from build123d import *

# Parameters (mm, degrees)
SZKIC2_W                    = 25.000000373
SZKIC2_H                    = 24
SZKIC2_R                    = 1.05
DODANIE_WYCI_GNI_CIE1_DEPTH = 5
SZKIC3_R                    = 1.05
WYTNIJ_WYCI_GNI_CIE1_DEPTH  = 36.134524248
SZKIC4_W                    = 2.5
SZKIC4_H                    = 6.5
SZKIC4_H_2                  = 12.5
WYTNIJ_WYCI_GNI_CIE2_DEPTH  = 36.134524248
ZAOKR_GLENIE5_R             = 2.5


with BuildPart() as part:
    # Szkic2 → Dodanie-wyciągnięcie1 (new body)
    with BuildSketch(Plane.XY):
        with Locations((12.381142653, 12.175085843)):
            Rectangle(SZKIC2_W, SZKIC2_H)
        with Locations((22.881142652, 22.175085947)):
            Circle(SZKIC2_R, mode=Mode.SUBTRACT)
        with Locations((22.881142652, 8.175085947)):
            Circle(SZKIC2_R, mode=Mode.SUBTRACT)
        with Locations((1.881142652, 22.175085947)):
            Circle(SZKIC2_R, mode=Mode.SUBTRACT)
        with Locations((1.881142652, 8.175085947)):
            Circle(SZKIC2_R, mode=Mode.SUBTRACT)
    extrude(amount=DODANIE_WYCI_GNI_CIE1_DEPTH)

    # Szkic3 → Wytnij-wyciągnięcie1 (cut, through all)
    with BuildSketch(Plane(origin=(24.881142839, 0, 0), x_dir=(0, 0, -1), z_dir=(1, 0, 0))):
        with Locations((-2.5, 15.175085843)):
            Circle(SZKIC3_R)
    extrude(amount=-WYTNIJ_WYCI_GNI_CIE1_DEPTH, mode=Mode.SUBTRACT)

    # Szkic4 → Wytnij-wyciągnięcie2 (cut, through all)
    with BuildSketch(Plane.ZY.offset(0.118857534)):
        with Locations((1.25, 20.925085843)):
            Rectangle(SZKIC4_W, SZKIC4_H)
        with Locations((1.25, 6.425085843)):
            Rectangle(SZKIC4_W, SZKIC4_H_2)
    extrude(amount=-WYTNIJ_WYCI_GNI_CIE2_DEPTH, mode=Mode.SUBTRACT)

    # Zaokrąglenie5
    zaokr_glenie5_edges = [part.edges().sort_by_distance(p)[0] for p in [
        (12.381142652, 12.675085843, 0),
        (12.381142652, 17.675085843, 0),
    ]]
    fillet(zaokr_glenie5_edges, radius=ZAOKR_GLENIE5_R - 0.0001)  # a hair under: the kernel refuses the full size


solid = part.part
The model under review builds one solid part; all positions refer to its coordinate system, in mm. A direction names the side the tool comes from. Round coordinates to 2 decimals unless told otherwise and drop trailing zeros. Write each loop counter-clockwise with the first axis right and the second up, starting at its lowest first coordinate (ties: lowest second). Pieces come first, ordered by that corner, then holes. Notation, with made-up numbers: (43, 57.25) - (80, 57.25) arc R21 cw to (80, 72.25) - close; hole circle Ø11 at (-2, 31). An arc over 180 degrees is marked (long way). One line per item, written item: value. Start each with the question number.
1. Consider section B-B on z = 3.15. Write out the cut boundary in (x, y).
2. Consider section A-A on y = 8.5. Write out the cut boundary in (x, z), and give its area (3 significant figures).
3. Clearance check with flat-ended pins moving along their axes: P1, Ø3.5, axis at x = 22.88, y = 22.18, coming from the -Z side; P2, Ø1.3, axis at y = 15.18, z = 2.5, coming from the -X side; P3, Ø4, axis at x = 8.5, y = 18, coming from the -Z side. State where each tip first meets the part, or that it passes through.
4. The part is to be moulded in two halves that separate along X. For faces 1 (the face through (21.832, 8.221, 3.732)), 2 (the face through (12.56, 16.92, 0.71)), 3 (the face through (-0.119, 12, 4)), 4 (the face through (1.744, 23.216, 3.732)), say which applies: released by +X, released by -X, zero draft, split by the parting line, or undercut.
5. Consider section C-C on z = 4.7. Write out the cut boundary in (x, y), and give its area (3 significant figures).
6. Machinability: for faces 5 (the face through (12, 6, 2.5)), 6 (the face through (22.744, 23.216, 3.732)), 7 (the face through (12, 21, 2.5)), which of the approach directions +Z, -Z, +X, -X, +Y, -Y give a long, thin tool a straight path to every point of the face, cutting with its end or side? Answer none if there is none.
7. To check wall thickness, follow L1, parallel to X at y = 7.75, z = 3.1; L2, parallel to Z at x = 8.5, y = 21.75; L3, parallel to Y at x = 24, z = 2.9. State the ranges of each line that lie inside material, in increasing order. Write a range as from..to.
Checks:
1. outline: (-0.12, 0.18) - (24.88, 0.18) - (24.88, 14.35) - (-0.12, 14.35) - close; (-0.12, 16) - (24.88, 16) - (24.88, 24.18) - (-0.12, 24.18) - close; hole circle Ø2.1 at (1.88, 8.18); hole circle Ø2.1 at (1.88, 22.18); hole circle Ø2.1 at (22.88, 8.18); hole circle Ø2.1 at (22.88, 22.18)
2. outline: (-0.12, 2.5) - (0.88, 2.5) - (0.88, 5) - (-0.12, 5) - close; (2.88, 2.5) - (21.88, 2.5) - (21.88, 5) - (2.88, 5) - close; (23.88, 2.5) - (24.88, 2.5) - (24.88, 5) - (23.88, 5) - close
2. area: 52.5 mm^2
3. P1: stops at z = 2.5
3. P2: passes through
3. P3: stops at z = 0.14
4. face 1: undercut
4. face 2: zero draft
4. face 3: released by -X
4. face 4: undercut
5. outline: (-0.12, 0.18) - (24.88, 0.18) - (24.88, 24.18) - (-0.12, 24.18) - close; hole circle Ø2.1 at (1.88, 8.18); hole circle Ø2.1 at (1.88, 22.18); hole circle Ø2.1 at (22.88, 8.18); hole circle Ø2.1 at (22.88, 22.18)
5. area: 586 mm^2
6. face 5: -Z, +X, -X, -Y
6. face 6: +Z, -Z
6. face 7: -Z, +X, -X, +Y
7. L1: x = -0.12..0.92, 2.84..21.92, 23.84..24.88
7. L2: z = 2.5..5
7. L3: y = 0.18..14.2, 16.15..24.18
